from build123d import *

# Parameters (mm, degrees)
F0_W     = 15
F0_H     = 15
F1_DEPTH = 15
F2_R     = 4.955
F3_DEPTH = 15.001
F4_R     = 4.955
F5_DEPTH = 30.001


with BuildPart() as f1:
    # F0 (on Top) → F1 (new body)
    with BuildSketch(Plane.XY):
        with Locations((-15, 0)):
            Rectangle(F0_W, F0_H)
        Rectangle(F0_W, F0_H)
        with Locations((15, 0)):
            Rectangle(F0_W, F0_H)
        with Locations((0, 15)):
            Rectangle(F0_W, F0_H)
        with Locations((0, -15)):
            Rectangle(F0_W, F0_H)
    extrude(amount=F1_DEPTH)

    # F2 (on face) → F3 (cut, through all)
    with BuildSketch(Plane.XY.offset(15)):
        with Locations((0, -15)):
            Circle(F2_R)
        with Locations((0, 15)):
            Circle(F2_R)
    extrude(amount=-F3_DEPTH, mode=Mode.SUBTRACT)

    # F4 (on face) → F5 (cut, through all)
    with BuildSketch(Plane(origin=(0, 7.5, 0), x_dir=(-1, 0, 0), z_dir=(0, 1, 0))):
        with Locations((15, 7.5)):
            Circle(F4_R)
        with Locations((-15, 7.5)):
            Circle(F4_R)
    extrude(amount=-F5_DEPTH, mode=Mode.SUBTRACT)


solid = f1.part
Could you check a few things on this model? Use its own coordinates, in mm. A direction names the side the tool comes from. Coordinates: 2 decimals unless noted, no trailing zeros. Order: outer loops, then holes, each group sorted by start corner. A loop starts at its lowest first (then second) coordinate and runs counter-clockwise, first axis right, second up.
Q1. Suppose I cut it at C-C on y = 3.5. Please give me the cut outline in (x, z) (3 decimals).
Q2. Suppose I cut it at A-A on z = 7.5. Please give me the cut outline in (x, y) (3 decimals), and give its area (3 significant figures).
Q3. Suppose I cut it at D-D on x = 0. Please give me the cut outline in (y, z) (3 decimals).
Q4. Will these pins go through, and if not, where does the flat tip stop? pin 1 (5 mm diameter, centred on y = -16.5, z = 13, fed in from -X); pin 2 (7.5 mm diameter, centred on x = 16, z = 4, fed in from +Y).
Q5. Suppose I cut it at B-B on x = 15. Please give me the cut outline in (y, z) (3 decimals).
Q6. Thinking about a two-plate mould opening in Y: for faces 4 (the flat face through (0, 22.5, 7)), 5 (the cylindrical face through (2.66, -10.82, 7.6)), 6 (the flat face through (22.5, 0, 7)), which applies, released by +Y, released by -Y, zero draft, split by the parting line, or undercut?
Q7. Please list where these lines run through material, in increasing order: L1, parallel to Z at x = 15, y = -4.25 (3 decimals); L2, parallel to Y at x = 0, z = 8.5 (3 decimals); L3, parallel to X at y = -2, z = 3.5.
Q8. Which directions (+Z, -Z, +X, -X, +Y, -Y) give clear straight access to the entire face, cutting with the end or side of a thin tool? Please do faces 1 (the flat face through (7.5, 15, 7)), 2 (the flat face through (-7.5, -15, 7)), 3 (the flat face through (15, -7.5, 2)).
Answer:
1. outline: (-22.5, 0) - (22.5, 0) - (22.5, 15) - (-22.5, 15) - close; hole circle Ø9.91 at (-15, 7.5); hole circle Ø9.91 at (15, 7.5)
2. outline: (-22.5, -7.5) - (-19.955, -7.5) - (-19.955, 7.5) - (-22.5, 7.5) - close; (-10.045, -7.5) - (-7.5, -7.5) - (-7.5, -22.5) - (7.5, -22.5) - (7.5, -7.5) - (10.045, -7.5) - (10.045, 7.5) - (7.5, 7.5) - (7.5, 22.5) - (-7.5, 22.5) - (-7.5, 7.5) - (-10.045, 7.5) - close; (19.955, -7.5) - (22.5, -7.5) - (22.5, 7.5) - (19.955, 7.5) - close; hole circle Ø9.91 at (0, -15); hole circle Ø9.91 at (0, 15)
2. area: 673 mm2
3. outline: (-22.5, 0) - (-19.955, 0) - (-19.955, 15) - (-22.5, 15) - close; (-10.045, 0) - (10.045, 0) - (10.045, 15) - (-10.045, 15) - close; (19.955, 0) - (22.5, 0) - (22.5, 15) - (19.955, 15) - close
4. pin 1: stops at x = -7.5
4. pin 2: stops at y = 7.5
5. outline: (-7.5, 0) - (7.5, 0) - (7.5, 2.545) - (-7.5, 2.545) - close; (-7.5, 12.455) - (7.5, 12.455) - (7.5, 15) - (-7.5, 15) - close
6. face 4: released by +Y
6. face 5: undercut
6. face 6: zero draft
7. L1: z = 0 to 2.545, 12.455 to 15
7. L2: y = -22.5 to -19.955, -10.045 to 10.045, 19.955 to 22.5
7. L3: x = -22.5 to -17.92, -12.08 to 12.08, 17.92 to 22.5
8. face 1: +Z, -Z, +X, +Y
8. face 2: +Z, -Z, -X, -Y
8. face 3: +Z, -Z, +X, -Y
